```python
from build123d import *

# Parameters (mm, degrees)
BOSS_EXTRUDE1_DEPTH = 27.800000026
SKETCH2_R           = 1.8288
CUT_EXTRUDE1_DEPTH  = 34.097129807


with BuildPart() as part:
    # Sketch1 → Boss-Extrude1 (new, symmetric)
    with BuildSketch(Plane.XY):
        Polygon((0, 12.7), (0, 0), (12.7, 0), (12.7, 3.175), (3.175, 3.175), (3.175, 12.7), align=None)
    extrude(amount=BOSS_EXTRUDE1_DEPTH, both=True)

    # Sketch2 → Cut-Extrude1 (cut, through all)
    with BuildSketch(Plane.ZY):
        with Locations((12.7, 6.35)):
            Circle(SKETCH2_R)
        with Locations((-12.7, 6.35)):
            Circle(SKETCH2_R)
    extrude(amount=-CUT_EXTRUDE1_DEPTH, mode=Mode.SUBTRACT)


solid = part.part
```
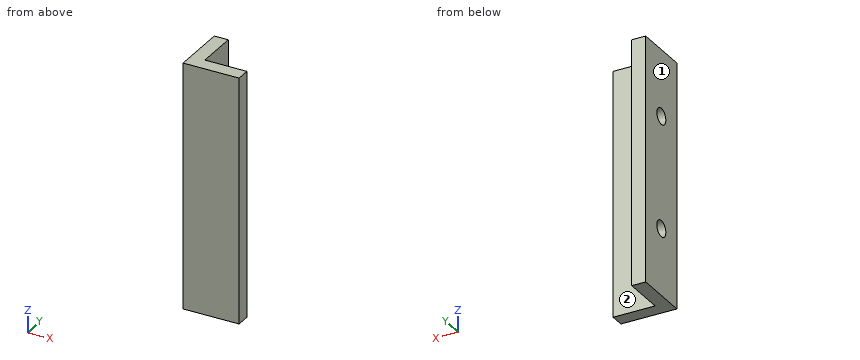
Part model, mm, in its own coordinate system. Face numbers are marked on the shaded views. A direction names the side the tool comes from. Coordinates: 2 decimals unless noted, no trailing zeros. Order: outer loops, then holes, each group sorted by start corner. A loop starts at its lowest first (then second) coordinate and runs counter-clockwise, first axis right, second up. Notation, with made-up numbers: (82, 4) - (119, 4) arc R24 cw to (119, 17) - close; hole circle Ø9 at (33, 84.5). An arc over 180 degrees is marked (long way). Return JSON: item names as keys, results as strings. Group by question number.
Item 1: Cut at D-D (x = 7). List the corners of the cut face in (y, z) (3 decimals), plus the area to 3 significant figures.
Item 2: Pin check, flat tips, straight feed: pin 1 (5 mm diameter, centred on y = 6.35, z = -12.7, fed in from +X) (3 decimals); pin 2 (7.5 mm diameter, centred on x = 9.5, z = 8, fed in from +Y) (3 decimals). Stop position of each tip, or through.
Item 3: Cut at A-A (y = 6.35). List the corners of the cut face in (x, z) (3 decimals), plus the area to 3 significant figures.
Item 4: Cut at B-B (z = -12.7). List the corners of the cut face in (x, y) (3 decimals).
Item 5: Cut at C-C (z = 8.5). List the corners of the cut face in (x, y) (3 decimals).
Item 6: Which spindle directions (+Z, -Z, +X, -X, +Y, -Y) get a long thin tool onto all of the face, cutting with end or side? Do the marked faces 1 and 2. Say none if no direction does.
Item 7: Drill centre lines: probe 1 along Z at (x, y) = (1.5, 6.5); probe 2 along Y at (x, z) = (0.85, -12.7); probe 3 along Z at (x, y) = (2, 8). Where is each one in solid material? Low to high. Write a range as from..to.
Check values:
{
 "1": {"outline": "(0, -27.8) - (3.175, -27.8) - (3.175, 27.8) - (0, 27.8) - close", "area": "177 mm2"},
 "2": {"pin 1": "stops at x = 3.175", "pin 2": "stops at y = 3.175"},
 "3": {"outline": "(0, -27.8) - (3.175, -27.8) - (3.175, -14.529) - (0, -14.529) - close; (0, -10.871) - (3.175, -10.871) - (3.175, 10.871) - (0, 10.871) - close; (0, 14.529) - (3.175, 14.529) - (3.175, 27.8) - (0, 27.8) - close", "area": "153 mm2"},
 "4": {"outline": "(0, 0) - (12.7, 0) - (12.7, 3.175) - (3.175, 3.175) - (3.175, 4.521) - (0, 4.521) - close; (0, 8.179) - (3.175, 8.179) - (3.175, 12.7) - (0, 12.7) - close"},
 "5": {"outline": "(0, 0) - (12.7, 0) - (12.7, 3.175) - (3.175, 3.175) - (3.175, 12.7) - (0, 12.7) - close"},
 "6": {"face 1": "+Z, -Z, -X, +Y, -Y", "face 2": "+Z, -Z, +X, +Y"},
 "7": {"probe 1": "z = -27.8..-14.52, -10.88..10.88, 14.52..27.8", "probe 2": "y = 0..4.52, 8.18..12.7", "probe 3": "z = -27.8..-13.49, -11.91..11.91, 13.49..27.8"}
}
